```python
from build123d import *

# Parameters (mm, degrees)
BOSS_EXTRUDE1_DEPTH = 22.86
SKETCH2_W           = 22.86
SKETCH2_H           = 5.715
SKETCH2_H_2         = 3.175
BOSS_EXTRUDE2_DEPTH = 17.145
SKETCH3_W           = 22.86
SKETCH3_H           = 5.715
SKETCH3_H_2         = 3.175
BOSS_EXTRUDE3_DEPTH = 17.145
SKETCH4_W           = 17.51
SKETCH4_H           = 3.175
CUT_EXTRUDE1_DEPTH  = 13.97
SKETCH5_W           = 17.51
SKETCH5_H           = 3.175
CUT_EXTRUDE2_DEPTH  = 13.97
SKETCH6_R           = 1.5875
CUT_EXTRUDE3_DEPTH  = 8.89
FILLET1_R           = 8.255
FILLET2_R           = 10.16
FILLET3_R           = 1
FILLET4_R           = 5
FILLET5_R           = 2


with BuildPart() as part:
    # Sketch1 → Boss-Extrude1 (new body)
    with BuildSketch(Plane.XY):
        Polygon((22.733, 17.145), (9.779, 17.145), (9.779, 13.97), (19.558, 13.97), (19.558, 6.985), (22.733, 6.985), align=None)
        Polygon((9.779, 13.97), (9.779, 17.145), (-3.175, 17.145), (-3.175, 6.985), (0, 6.985), (0, 13.97), align=None)
    extrude(amount=BOSS_EXTRUDE1_DEPTH)

    # Sketch2 → Boss-Extrude2 (add)
    with BuildSketch(Plane.ZY.offset(3.175)):
        with Locations((11.43, 9.8425)):
            Rectangle(SKETCH2_W, SKETCH2_H)
        with Locations((11.43, 5.3975)):
            Rectangle(SKETCH2_W, SKETCH2_H_2)
    extrude(amount=BOSS_EXTRUDE2_DEPTH)

    # Sketch3 → Boss-Extrude3 (add)
    with BuildSketch(Plane(origin=(22.733, 0, 0), x_dir=(0, 0, -1), z_dir=(1, 0, 0))):
        with Locations((-11.43, 9.8425)):
            Rectangle(SKETCH3_W, SKETCH3_H)
        with Locations((-11.43, 5.3975)):
            Rectangle(SKETCH3_W, SKETCH3_H_2)
    extrude(amount=BOSS_EXTRUDE3_DEPTH)

    # Sketch4 → Cut-Extrude1 (cut)
    with BuildSketch(Plane.ZY.offset(-22.733)):
        with Locations((11.43, 5.3975)):
            Rectangle(SKETCH4_W, SKETCH4_H)
    extrude(amount=-CUT_EXTRUDE1_DEPTH, mode=Mode.SUBTRACT)

    # Sketch5 → Cut-Extrude2 (cut)
    with BuildSketch(Plane(origin=(-3.175, 0, 0), x_dir=(0, 0, -1), z_dir=(1, 0, 0))):
        with Locations((-11.43, 5.3975)):
            Rectangle(SKETCH5_W, SKETCH5_H)
    extrude(amount=-CUT_EXTRUDE2_DEPTH, mode=Mode.SUBTRACT)

    # Sketch6 → Cut-Extrude3 (cut)
    with BuildSketch(Plane(origin=(0, 12.7, 0), x_dir=(1, 0, 0), z_dir=(0, 1, 0))):
        with Locations(Location((29.9466, -11.43, 0), (0, 0, 270))):
            Circle(SKETCH6_R)
        with Locations(Location((-10.3886, -11.43, 0), (0, 0, 270))):
            Circle(SKETCH6_R)
    extrude(amount=-CUT_EXTRUDE3_DEPTH, mode=Mode.SUBTRACT)

    # Fillet1
    fillet1_edges = [part.edges().sort_by_distance(p)[0] for p in [
        (36.703, 5.3975, 2.675),
        (36.703, 5.3975, 20.185),
        (-17.145, 5.3975, 20.185),
        (-17.145, 5.3975, 2.675),
    ]]
    fillet(fillet1_edges, radius=FILLET1_R)

    # Fillet2
    fillet2_edges = [part.edges().sort_by_distance(p)[0] for p in [
        (-20.32, 8.255, 22.86),
        (-20.32, 8.255, 0),
        (39.878, 8.255, 22.86),
        (39.878, 8.255, 0),
    ]]
    fillet(fillet2_edges, radius=FILLET2_R)

    # Fillet3
    fillet3_edges = [part.edges().sort_by_distance(p)[0] for p in [
        (19.558, 13.97, 11.43),
        (0, 13.97, 11.43),
    ]]
    fillet(fillet3_edges, radius=FILLET3_R)

    # Fillet4
    # the kernel refuses this fillet: 5 mm, written as the material it takes off along each edge
    with BuildSketch(Plane(origin=(22.733, 17.145, -12.422755079), x_dir=(-1, 0, 0), z_dir=(0, 0, 1))) as fillet4_piece_1:
        with BuildLine():
            CenterArc((4.969102032, 5), FILLET4_R, 186.372964386, 83.627035614)
            Line((0, 4.445), (-0.099382041, 4.4339))
            ThreePointArc((-0.099382041, 4.4339), (-0.1, 2.2225), (-0.1, 0))
            Line((-0.1, 0), (0, -0.1))
            Line((0, -0.1), (4.969102032, -0.1))
            Line((4.969102032, -0.1), (4.969102032, 0))
        make_face()
    extrude(amount=47.705510158, mode=Mode.SUBTRACT)
    with BuildSketch(Plane(origin=(-3.175, 17.145, -12.422755079), x_dir=(0, -1, 0), z_dir=(0, 0, 1))) as fillet4_piece_2:
        with BuildLine():
            CenterArc((5, 4.969102032), FILLET4_R, 180, 83.627035614)
            Line((0, 4.969102032), (-0.1, 4.969102032))
            Line((-0.1, 4.969102032), (-0.1, 0))
            Line((-0.1, 0), (0, -0.1))
            ThreePointArc((0, -0.1), (2.2225, -0.1), (4.4339, -0.099382041))
            Line((4.4339, -0.099382041), (4.445, 0))
        make_face()
    extrude(amount=47.705510158, mode=Mode.SUBTRACT)

    # Fillet5
    fillet5_edges = [part.edges().sort_by_distance(p)[0] for p in [
        (-20.32, 12.7, 11.43),
        (-6.6675, 12.7, 0),
        (-6.6675, 12.7, 22.86),
        (-17.344204897, 12.7, 2.975795103),
        (-17.344204897, 12.7, 19.884204897),
        (26.2255, 12.7, 22.86),
        (26.2255, 12.7, 0),
        (39.878, 12.7, 11.43),
        (36.902204897, 12.7, 2.975795103),
        (36.902204897, 12.7, 19.884204897),
        (9.779, 17.145, 0),
        (9.779, 17.145, 22.86),
        (-1.539439629, 15.871593619, 0),
        (21.097439629, 15.871593619, 0),
        (-1.539439629, 15.871593619, 22.86),
        (21.097439629, 15.871593619, 22.86),
        (-3.175, 12.7, 11.43),
        (22.733, 12.7, 11.43),
    ]]
    fillet(fillet5_edges, radius=FILLET5_R)


solid = part.part
```
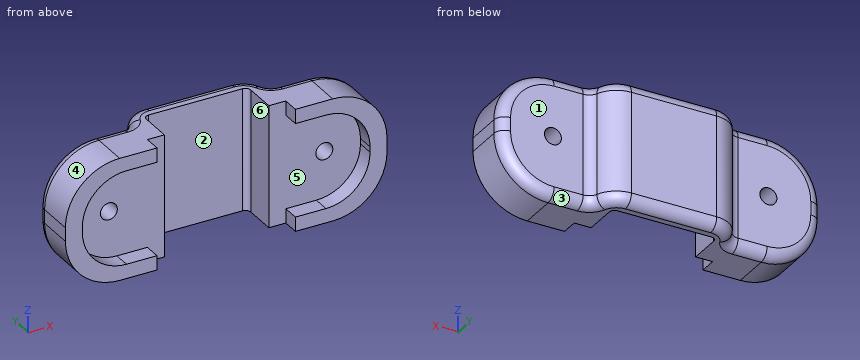
For this review, take the finished solid that the model builds, in its own axes (mm). Face numbers are marked on the shaded views. A direction names the side the tool comes from. Coordinates: 2 decimals unless noted, no trailing zeros. Loops run counter-clockwise (first coordinate to the right, second up) from the corner with the lowest first, then second, coordinate; pieces in that order, holes last.
1. Insertion check: P1, Ø3.5, axis at x = 29.95, z = 11.43, coming from the +Y side; P2, Ø5, axis at y = 11, z = 8, coming from the +X side; P3, Ø1, axis at x = -10.5, y = 12.5, coming from the +Z side; P4, Ø0.8, axis at y = 5.5, z = 1.5, coming from the -X side. Each pin has a flat end and moves straight along its axis. Give the tip position at first contact, or say it passes through.
2. Add section B-B, the plane y = 9. Give the boundary of the cut face in (x, z) (1 decimal).
3. Add section D-D, the plane x = 15. Give the boundary of the cut face in (y, z) (3 decimals), then the cut area to 3 significant figures.
4. Mouldability with a two-part tool opening along Z and no side actions: class the marked faces 4, 5 and 6 as +Z half, -Z half, draft (parallel to the pull), parting line (faces both ways), or undercut.
5. Add section A-A, the plane y = 5. Give the boundary of the cut face in (x, z) (3 decimals), then the cut area to 3 significant figures.
6. For the marked faces 1, 2 and 3, list the 3-axis set-ups (+Z, -Z, +X, -X, +Y, -Y) from which the entire face can be reached by the end or side of a thin tool; tool diameter is ignored.
7. For line 1 (X direction, y = 9.65, z = 11.43); line 2 (Y direction, x = 33, z = 7) (3 decimals); line 3 (Y direction, x = 8, z = 3) (3 decimals), list the stretches that pass through material, from the lowest coordinate up.
8. Add section C-C, the plane x = -7. Give the boundary of the cut face in (y, z) (3 decimals).
Result:
1. P1: stops at y = 12.7
1. P2: stops at x = 39.88
1. P3: stops at z = 22.37
1. P4: stops at x = -16.08
2. outline: (-20.3, 10.2) arc R10.2 ccw to (-10.2, 0) - (0, 0) - (0, 22.9) - (-10.2, 22.9) arc R10.2 ccw to (-20.3, 12.7) - close; (19.6, 0) - (29.7, 0) arc R10.2 ccw to (39.9, 10.2) - (39.9, 12.7) arc R10.2 ccw to (29.7, 22.9) - (19.6, 22.9) - close; hole circle Ø3.2 at (-10.4, 11.4); hole circle Ø3.2 at (29.9, 11.4)
3. outline: (13.97, 0) - (15.145, 0) arc R2 ccw to (17.145, 2) - (17.145, 20.86) arc R2 ccw to (15.145, 22.86) - (13.97, 22.86) - close
3. area: 70.9 mm2
4. face 4: +Z half
4. face 5: undercut
4. face 6: draft
5. outline: (-20.32, 10.16) arc R10.16 ccw to (-10.16, 0) - (-3.175, 0) - (-3.175, 2.675) - (-8.89, 2.675) arc R8.255 cw to (-17.145, 10.93) - (-17.145, 11.93) arc R8.255 cw to (-8.89, 20.185) - (-3.175, 20.185) - (-3.175, 22.86) - (-10.16, 22.86) arc R10.16 ccw to (-20.32, 12.7) - close; (22.733, 0) - (29.718, 0) arc R10.16 ccw to (39.878, 10.16) - (39.878, 12.7) arc R10.16 ccw to (29.718, 22.86) - (22.733, 22.86) - (22.733, 20.185) - (28.448, 20.185) arc R8.255 cw to (36.703, 11.93) - (36.703, 10.93) arc R8.255 cw to (28.448, 2.675) - (22.733, 2.675) - close
5. area: 265 mm2
6. face 1: +Z, -Z, +X, +Y
6. face 2: +Z, -Z, -Y
6. face 3: -Z, +X, +Y
7. line 1: x = -20.32 to -11.98, -8.8 to 0, 19.56 to 28.36, 31.53 to 39.88
7. line 2: y = 6.985 to 12.7
7. line 3: y = 13.97 to 17.145
8. outline: (3.81, 0) - (10.7, 0) arc R2 ccw to (12.7, 2) - (12.7, 20.86) arc R2 ccw to (10.7, 22.86) - (3.81, 22.86) - (3.81, 20.185) - (6.985, 20.185) - (6.985, 2.675) - (3.81, 2.675) - close
